Design review of the part built by this model. Coordinates are the model's own, in mm. Round coordinates to 2 decimals unless told otherwise and drop trailing zeros. Write each loop counter-clockwise with the first axis right and the second up, starting at its lowest first coordinate (ties: lowest second). Pieces come first, ordered by that corner, then holes. Notation, with made-up numbers: (6, -35) -> (61, -35) arc R28 cw to (61, 3) -> close; hole circle Ø10 at (-34.75, 47.5). An arc over 180 degrees is marked (long way). One line per question, with ' | ' between items. Start each with the question number.
1) Consider section C-C (x = 92.5). Give the boundary of the cut face in (y, z), then the cut area to 3 significant figures.
2) Consider section B-B (x = 54). Give the boundary of the cut face in (y, z).
3) For probe 1 along Y at (x, z) = (29, 2.4); probe 2 along X at (y, z) = (-0.5, 1.1); probe 3 along Y at (x, z) = (128, 1.2), list the stretches that pass through material, from the lowest coordinate up.
4) Consider section A-A (z = 1.65). Count the separate pieces of the cut face and the enclosed holes in it, then the cut area to 3 significant figures.
5) Insertion check: pin 1 Ø1.5 at (x, z) = (150.5, 2) entering from -Y; pin 2 Ø1.5 at (x, z) = (48, 1.5) entering from -Y; pin 3 Ø0.9 at (x, z) = (159.5, 2) entering from +Y; pin 4 Ø2.5 at (x, y) = (19, -33.75) entering from -Z (3 decimals). Each pin has a flat end and moves straight along its axis. Give the tip position at first contact, or say it passes through.
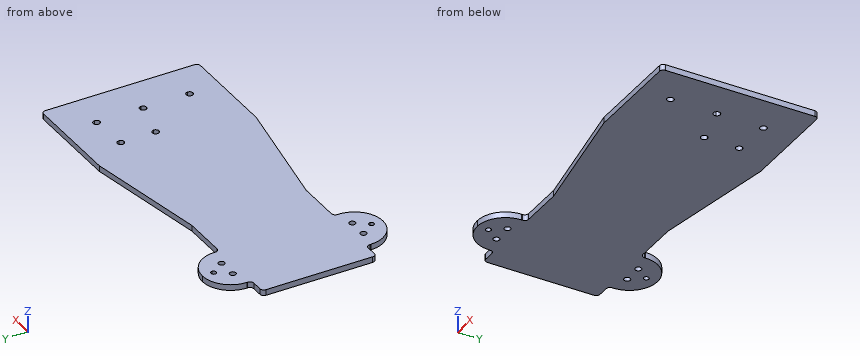
```python
from build123d import *

# Parameters (mm, degrees)
F0_R     = 1.6
F1_DEPTH = 3


with BuildPart() as f1:
    # F0 (on Top) → F1 (new body)
    with BuildSketch(Plane.XY):
        Polygon((63, 29.5), (63, 0), (127, 0), (127, 40.5), align=None)
        with BuildLine():
            Line((127, 0), (63, 0))
            Line((63, 0), (24, 0))
            Line((24, 0), (24, -39.4))
            ThreePointArc((24, -39.4), (24.954594, -39.795406), (25.35, -40.75))
            ThreePointArc((25.35, -40.75), (24.954594, -41.704594), (24, -42.1))
            Line((24, -42.1), (24, -46.5))
            ThreePointArc((24, -46.5), (34.253048, -42.253048), (38.5, -32))
            Line((38.5, -32), (38.5, -31.5))
            ThreePointArc((38.5, -31.5), (39.085786, -30.085786), (40.5, -29.5))
            Line((40.5, -29.5), (63, -29.5))
            Line((63, -29.5), (127, -40.5))
            Line((127, -40.5), (139, -40.5))
            Line((139, -40.5), (139, 0))
            Line((139, 0), (127, 0))
        make_face()
        with Locations((29, -33.75)):
            Circle(F0_R, mode=Mode.SUBTRACT)
        with BuildLine():
            Line((24, 0), (63, 0))
            Line((63, 0), (63, 29.5))
            Line((63, 29.5), (40.5, 29.5))
            ThreePointArc((40.5, 29.5), (39.085786, 30.085786), (38.5, 31.5))
            Line((38.5, 31.5), (38.5, 32))
            Line((38.5, 32), (24, 32))
            Line((24, 32), (24, 0))
        make_face()
        with BuildLine():
            Line((127, 40.5), (127, 0))
            Line((127, 0), (139, 0))
            Line((139, 0), (139, 2.75))
            ThreePointArc((139, 2.75), (137.25, 4.5), (139, 6.25))
            Line((139, 6.25), (139, 20.75))
            ThreePointArc((139, 20.75), (137.25, 22.5), (139, 24.25))
            Line((139, 24.25), (139, 40.5))
            Line((139, 40.5), (127, 40.5))
        make_face()
        with BuildLine():
            Line((24, -39.4), (24, 0))
            Line((24, 0), (0, 0))
            Line((0, 0), (0, -27.5))
            ThreePointArc((0, -27.5), (0.585786, -28.914214), (2, -29.5))
            Line((2, -29.5), (7.5, -29.5))
            ThreePointArc((7.5, -29.5), (8.914214, -30.085786), (9.5, -31.5))
            Line((9.5, -31.5), (9.5, -32))
            ThreePointArc((9.5, -32), (13.746952, -42.253048), (24, -46.5))
            Line((24, -46.5), (24, -42.1))
            ThreePointArc((24, -42.1), (22.65, -40.75), (24, -39.4))
        make_face()
        with Locations((19, -33.75)):
            Circle(F0_R, mode=Mode.SUBTRACT)
        with BuildLine():
            Line((0, 0), (24, 0))
            Line((24, 0), (24, 32))
            Line((24, 32), (9.5, 32))
            Line((9.5, 32), (9.5, 31.5))
            ThreePointArc((9.5, 31.5), (8.914214, 30.085786), (7.5, 29.5))
            Line((7.5, 29.5), (2, 29.5))
            ThreePointArc((2, 29.5), (0.585786, 28.914214), (0, 27.5))
            Line((0, 27.5), (0, 0))
        make_face()
        with BuildLine():
            Line((139, 2.75), (139, 0))
            Line((139, 0), (157.322949, 0))
            ThreePointArc((157.322949, 0), (157.954175, 0.903122), (159, 1.25))
            Line((159, 1.25), (159, 21.75))
            ThreePointArc((159, 21.75), (157.25, 23.5), (159, 25.25))
            Line((159, 25.25), (159, 40.5))
            Line((159, 40.5), (139, 40.5))
            Line((139, 40.5), (139, 24.25))
            ThreePointArc((139, 24.25), (140.237437, 23.737437), (140.75, 22.5))
            ThreePointArc((140.75, 22.5), (140.237437, 21.262563), (139, 20.75))
            Line((139, 20.75), (139, 6.25))
            ThreePointArc((139, 6.25), (140.237437, 5.737437), (140.75, 4.5))
            ThreePointArc((140.75, 4.5), (140.237437, 3.262563), (139, 2.75))
        make_face()
        with BuildLine():
            Line((157.322949, 0), (139, 0))
            Line((139, 0), (139, -40.5))
            Line((139, -40.5), (159, -40.5))
            Line((159, -40.5), (159, -26.25))
            ThreePointArc((159, -26.25), (157.25, -24.5), (159, -22.75))
            Line((159, -22.75), (159, -2.25))
            ThreePointArc((159, -2.25), (157.596878, -1.545825), (157.322949, 0))
        make_face()
        with BuildLine():
            Line((24, 39.4), (24, 32))
            Line((24, 32), (38.5, 32))
            ThreePointArc((38.5, 32), (34.253048, 42.253048), (24, 46.5))
            Line((24, 46.5), (24, 42.1))
            ThreePointArc((24, 42.1), (24.954594, 41.704594), (25.35, 40.75))
            ThreePointArc((25.35, 40.75), (24.954594, 39.795406), (24, 39.4))
        make_face()
        with Locations((29, 33.75)):
            Circle(F0_R, mode=Mode.SUBTRACT)
        with BuildLine():
            Line((9.5, 32), (24, 32))
            Line((24, 32), (24, 39.4))
            ThreePointArc((24, 39.4), (22.65, 40.75), (24, 42.1))
            Line((24, 42.1), (24, 46.5))
            ThreePointArc((24, 46.5), (13.746952, 42.253048), (9.5, 32))
        make_face()
        with Locations((19, 33.75)):
            Circle(F0_R, mode=Mode.SUBTRACT)
        with BuildLine():
            Line((159, 21.75), (159, 1.25))
            ThreePointArc((159, 1.25), (160.045825, 0.903122), (160.677051, 0))
            Line((160.677051, 0), (179, 0))
            Line((179, 0), (179, 38.5))
            ThreePointArc((179, 38.5), (178.414214, 39.914214), (177, 40.5))
            Line((177, 40.5), (159, 40.5))
            Line((159, 40.5), (159, 25.25))
            ThreePointArc((159, 25.25), (160.237437, 24.737437), (160.75, 23.5))
            ThreePointArc((160.75, 23.5), (160.237437, 22.262563), (159, 21.75))
        make_face()
        with BuildLine():
            ThreePointArc((160.75, -0.5), (160.237437, -1.737437), (159, -2.25))
            Line((159, -2.25), (159, -22.75))
            ThreePointArc((159, -22.75), (160.237437, -23.262563), (160.75, -24.5))
            ThreePointArc((160.75, -24.5), (160.237437, -25.737437), (159, -26.25))
            Line((159, -26.25), (159, -40.5))
            Line((159, -40.5), (177, -40.5))
            ThreePointArc((177, -40.5), (178.414214, -39.914214), (179, -38.5))
            Line((179, -38.5), (179, 0))
            Line((179, 0), (160.677051, 0))
            ThreePointArc((160.677051, 0), (160.731667, -0.247353), (160.75, -0.5))
        make_face()
    extrude(amount=F1_DEPTH)


solid = f1.part
```
From the geometry:
1) outline: (-34.57, 0) -> (34.57, 0) -> (34.57, 3) -> (-34.57, 3) -> close | area: 207 mm2
2) outline: (-29.5, 0) -> (29.5, 0) -> (29.5, 3) -> (-29.5, 3) -> close
3) probe 1: y = -45.61 to -35.35, -32.15 to 32.15, 35.35 to 45.61 | probe 2: x = 0 to 157.25, 160.75 to 179 | probe 3: y = -40.5 to 40.5
4) separate pieces: 1 | enclosed holes: 11 | area: 13,100 mm2
5) pin 1: stops at y = -40.5 | pin 2: stops at y = -29.5 | pin 3: stops at y = 40.5 | pin 4: passes through
